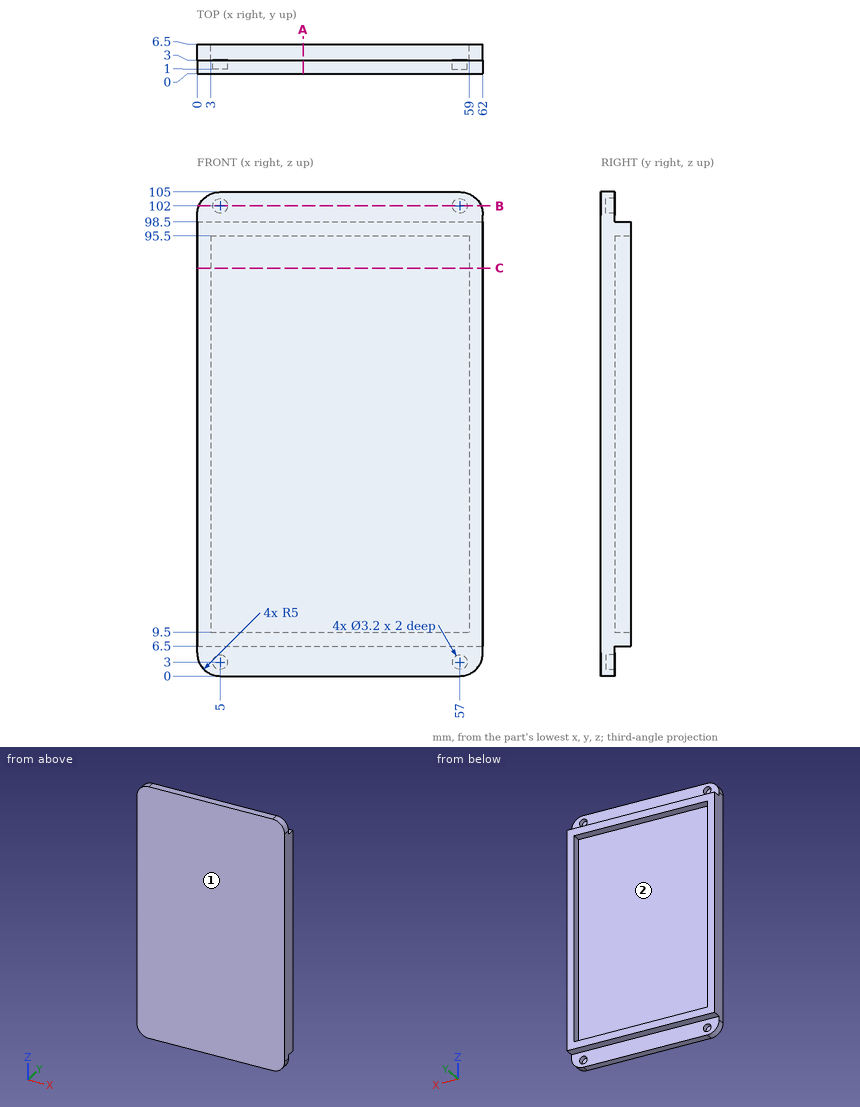
Source: three-view drawing plus pictorial views. Frame: mm from the lowest corner of the part. Give positions to 0.01 mm unless a question says otherwise; leave off trailing zeros. Order: outer loops, then holes, each group sorted by start corner. A loop starts at its lowest first (then second) coordinate and runs counter-clockwise, first axis right, second up. Notation, with made-up numbers: M 64.5,47 L 109.5,47 A25 cw 109.5,80 Z; hole C 36,20.25 d3. An arc over 180 degrees is marked long. One line per question, with ' | ' between items.
1) Contact query for flat-ended pins moving along their axis: P1, Ø1, axis at x = 26, y = 5, coming from the -Z side; P2, Ø1.6, axis at x = 57, z = 103, coming from the +Y side; P3, Ø1.6, axis at x = 57, z = 3, coming from the +Y side. Output: stop coordinate, or through.
Filled in:
P1: stops at z = 6.5 | P2: stops at y = 3 | P3: stops at y = 1
2) Section A-A on x = 23. Output: boundary loops of the cut face in (y, z).
Filled in:
outline: M 0,0 L 3,0 L 3,6.5 L 6.5,6.5 L 6.5,9.5 L 3,9.5 L 3,95.5 L 6.5,95.5 L 6.5,98.5 L 3,98.5 L 3,105 L 0,105 Z
3) Section B-B on z = 102. Output: boundary loops of the cut face in (x, y), and give its area (3 significant figures).
Filled in:
outline: M 0.42,0 L 61.58,0 L 61.58,3 L 58.6,3 L 58.6,1 L 55.4,1 L 55.4,3 L 6.6,3 L 6.6,1 L 3.4,1 L 3.4,3 L 0.42,3 Z | area: 171 mm2
4) Draft query along X for the marked faces 1 and 2. Return one class per face: pulls with the +X half, pulls with the -X half, needs draft (parallel to the pull), parting line crosses it, or undercut.
Filled in:
face 1: needs draft | face 2: undercut
5) Section C-C on z = 88.5. Output: boundary loops of the cut face in (x, y), and give its area (3 significant figures).
Filled in:
outline: M 0,0 L 62,0 L 62,6.5 L 59,6.5 L 59,3 L 3,3 L 3,6.5 L 0,6.5 Z | area: 207 mm2
6) Ray query, L1, parallel to Z at x = 49, y = 6.25; L2, parallel to X at y = 5, z = 42; L3, parallel to X at y = 2, z = 3. Return the intervals inside material, ascending.
Filled in:
L1: z = 6.5 to 9.5, 95.5 to 98.5 | L2: x = 0 to 3, 59 to 62 | L3: x = 0.42 to 3.4, 6.6 to 55.4, 58.6 to 61.58
